Can you work these out from the drawing? Everything is in mm from the part's minimum corner. Coordinates: 2 decimals unless noted, no trailing zeros. Order: outer loops, then holes, each group sorted by start corner. A loop starts at its lowest first (then second) coordinate and runs counter-clockwise, first axis right, second up. Notation, with made-up numbers: (-12, 84.5) - (41, 84.5) arc R21 cw to (41, 109.5) - close; hole circle Ø8 at (84, -36.5). An arc over 180 degrees is marked (long way). Use a Markdown table: item, result. Add a question column.
(1) I want a section at A-A (x = 8). List the corners of the cut face in (y, z) for me, and give its area (3 significant figures).
(2) We'd pull the mould along X, two halves only. Please class the marked faces 1, 2 and 3: pulls with the +X half, pulls with the -X half, needs draft (parallel to the pull), parting line crosses it, or undercut.
(3) If I drill on L1, parallel to Z at x = 8, y = 3.6; L2, parallel to X at y = 1.35, z = 32.5; L3, parallel to Z at x = 6, y = 0.5, over which ranges is the centre line in solid material (lowest first)? Write a range as [from, to].
(4) I want a section at B-B (y = 3.7). List the corners of the cut face in (x, z) for me.
(5) I want a section at D-D (z = 9.5). List the corners of the cut face in (x, y) for me.
(6) For pin 1 Ø6 at (x, z) = (8, 9) entering from +Y, with a flat end and sliding along its axis, tell me the tip position at first contact or that it passes through.
(7) I want a section at C-C (z = 51). List the corners of the cut face in (x, y) for me, and give its area (3 significant figures).
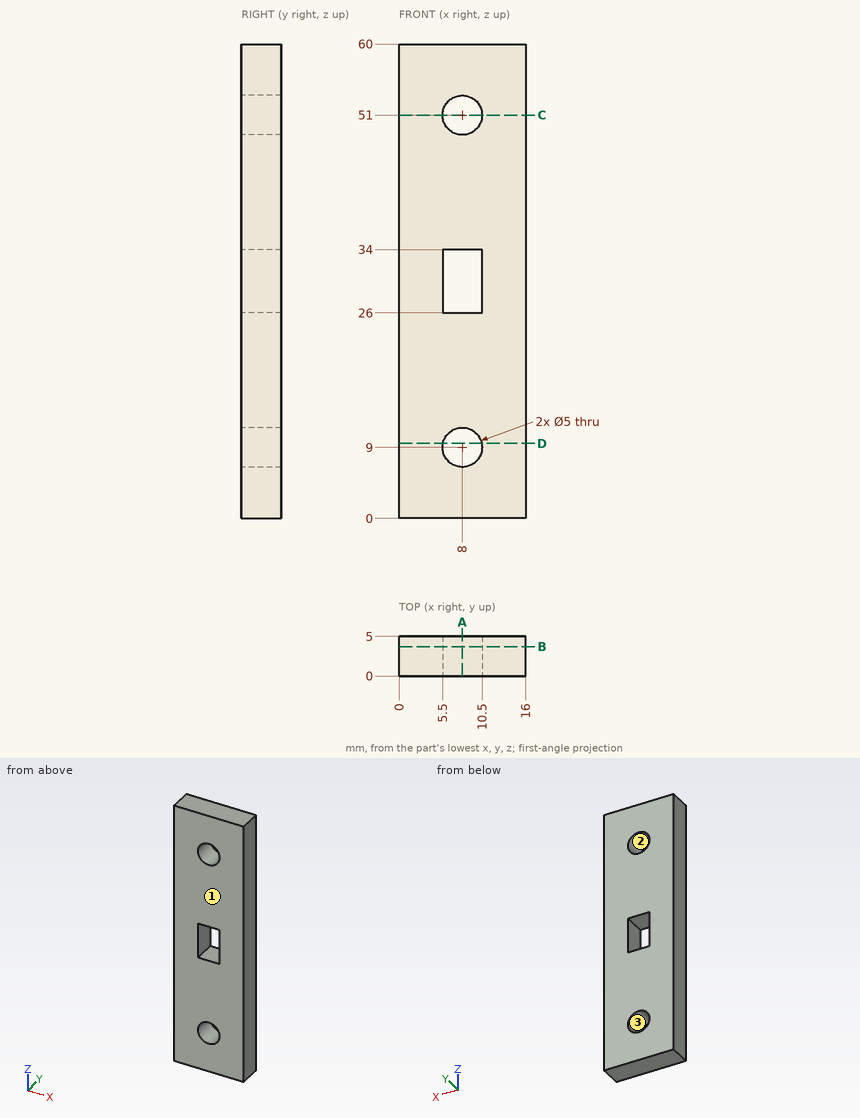
Answers follow:
| question | item | result |
|---|---|---|
| 1 | outline | (0, 0) - (5, 0) - (5, 6.5) - (0, 6.5) - close; (0, 11.5) - (5, 11.5) - (5, 26) - (0, 26) - close; (0, 34) - (5, 34) - (5, 48.5) - (0, 48.5) - close; (0, 53.5) - (5, 53.5) - (5, 60) - (0, 60) - close |
| 1 | area | 210 mm² |
| 2 | face 1 | needs draft |
| 2 | face 2 | undercut |
| 2 | face 3 | undercut |
| 3 | L1 | z = [0, 6.5], [11.5, 26], [34, 48.5], [53.5, 60] |
| 3 | L2 | x = [0, 5.5], [10.5, 16] |
| 3 | L3 | z = [0, 7.5], [10.5, 26], [34, 49.5], [52.5, 60] |
| 4 | outline | (0, 0) - (16, 0) - (16, 60) - (0, 60) - close; hole circle Ø5 at (8, 9); hole (5.5, 26) - (10.5, 26) - (10.5, 34) - (5.5, 34) - close; hole circle Ø5 at (8, 51) |
| 5 | outline | (0, 0) - (5.55, 0) - (5.55, 5) - (0, 5) - close; (10.45, 0) - (16, 0) - (16, 5) - (10.45, 5) - close |
| 6 | pin 1 | stops at y = 5 |
| 7 | outline | (0, 0) - (5.5, 0) - (5.5, 5) - (0, 5) - close; (10.5, 0) - (16, 0) - (16, 5) - (10.5, 5) - close |
| 7 | area | 55.0 mm² |
